from build123d import *

# Parameters (mm, degrees)
F1_DEPTH    = 112
F2_R        = 25
F3_DEPTH    = 185
F2_R_2      = 31.5
F5_DEPTH    = 184
F6_DEPTH    = 95
F7_W        = 48
F7_H        = 100
F8_DEPTH    = 159
F9_R        = 5.5
F10_DEPTH   = 39.1
F9_R_2      = 1.5
F11_DEPTH   = 154.4
F12_SIZE2   = 32
F12_SIZE    = 20
F12_2_SIZE2 = 32
F12_2_SIZE  = 20


with BuildPart() as f1:
    # F0 (on Front) → F1 (new body)
    with BuildSketch(Plane.XZ):
        with BuildLine():
            ThreePointArc((-59.7957043946, -22.8214863997), (-55.1094128936, -34.1351948987), (-43.7957043946, -38.8214863997))
            Line((-43.7957043946, -38.8214863997), (19.2042956054, -38.8214863997))
            ThreePointArc((19.2042956054, -38.8214863997), (30.5180041044, -34.1351948987), (35.2042956054, -22.8214863997))
            Line((35.2042956054, -22.8214863997), (35.2042956054, 103.1785136003))
            Line((35.2042956054, 103.1785136003), (29.2042956054, 103.1785136003))
            Line((29.2042956054, 103.1785136003), (29.2042956054, 87.1785136003))
            Line((29.2042956054, 87.1785136003), (29.2042956054, -23.8214863997))
            ThreePointArc((29.2042956054, -23.8214863997), (26.5682566361, -30.1854474304), (20.2042956054, -32.8214863997))
            Line((20.2042956054, -32.8214863997), (-44.7957043946, -32.8214863997))
            ThreePointArc((-44.7957043946, -32.8214863997), (-51.1596654253, -30.1854474304), (-53.7957043946, -23.8214863997))
            Line((-53.7957043946, -23.8214863997), (-53.7957043946, 86.1785136003))
            Line((-53.7957043946, 86.1785136003), (-59.7957043946, 86.1785136003))
            Line((-59.7957043946, 86.1785136003), (-59.7957043946, -22.8214863997))
        make_face()
    extrude(amount=F1_DEPTH)

    # F2 (on face) → F3 (cut)
    with BuildSketch(Plane.YZ.offset(35.2042956054)):
        with Locations((-56, 47.1785136003)):
            Circle(F2_R)
    extrude(amount=-F3_DEPTH, mode=Mode.SUBTRACT)

    # F2 (on face) → F5 (cut)
    with BuildSketch(Plane.YZ.offset(35.2042956054)):
        with Locations((-56, 47.1785136003)):
            Circle(F2_R_2)
        with Locations((-56, 47.1785136003)):
            Circle(F2_R, mode=Mode.SUBTRACT)
    extrude(amount=-F5_DEPTH, mode=Mode.SUBTRACT)

    # F2 (on face) → F6 (join)
    with BuildSketch(Plane.YZ.offset(35.2042956054)):
        with Locations((-56, 47.1785136003)):
            Circle(F2_R_2)
        with Locations((-56, 47.1785136003)):
            Circle(F2_R, mode=Mode.SUBTRACT)
    extrude(amount=-F6_DEPTH)

    # F7 (on offset) → F8 (cut)
    with BuildSketch(Plane.XZ.offset(137)):
        with Locations((-11.7957043946, 29.1785136003)):
            Rectangle(F7_W, F7_H)
    extrude(amount=-F8_DEPTH, mode=Mode.SUBTRACT)

    # F9 (on face) → F10 (cut)
    with BuildSketch(Plane.YZ.offset(35.2042956054)):
        with Locations((-83, 92.1785136003)):
            Circle(F9_R)
        with Locations((-29, 92.1785136003)):
            Circle(F9_R)
        with Locations((-95, 7.1785136003)):
            Circle(F9_R)
        with Locations((-17, 7.1785136003)):
            Circle(F9_R)
    extrude(amount=-F10_DEPTH, mode=Mode.SUBTRACT)

    # F9 (on face) → F11 (cut)
    with BuildSketch(Plane.YZ.offset(35.2042956054)):
        with Locations((-31.751288694, 33.2468845546)):
            Circle(F9_R_2)
        with Locations((-80.248711306, 33.2468845546)):
            Circle(F9_R_2)
        with BuildLine():
            ThreePointArc((-56, 73.7468845546), (-54.9393398282, 74.1862243828), (-54.5, 75.2468845546))
            ThreePointArc((-54.5, 75.2468845546), (-57.0606601718, 76.3075447264), (-56, 73.7468845546))
        make_face()
    extrude(amount=-F11_DEPTH, mode=Mode.SUBTRACT)

    # F12
    f12_edges = [f1.edges().sort_by_distance(p)[0] for p in [
        (-56.795704, 0, 86.178514),
        (-56.795704, -112, 86.178514),
    ]]
    f12_side = f1.faces().sort_by_distance((-56.795704, -56, 86.178514))[0]
    chamfer(f12_edges, length=F12_SIZE, length2=F12_SIZE2, reference=f12_side)

    # F12#2
    f12_2_edges = [f1.edges().sort_by_distance(p)[0] for p in [
        (32.204296, 0, 103.178514),
        (32.204296, -112, 103.178514),
    ]]
    f12_2_side = f1.faces().sort_by_distance((32.204296, -56, 103.178514))[0]
    chamfer(f12_2_edges, length=F12_2_SIZE, length2=F12_2_SIZE2, reference=f12_2_side)


solid = f1.part
Source: CAD feature listing. Evaluate the final solid. Frame: model axes, mm. A direction names the side the tool comes from. Coordinates: 2 decimals unless noted, no trailing zeros. Loops run counter-clockwise (first coordinate to the right, second up) from the corner with the lowest first, then second, coordinate; pieces in that order, holes last. Notation, with made-up numbers: (79, 27.5) - (99, 27.5) arc R11 cw to (99, 41.5) - close; hole circle Ø9 at (30.25, -17.5). An arc over 180 degrees is marked (long way). Return JSON: item names as keys, results as strings.
Q1. Section C-C, the plane y = -95. Return loops of the section in (x, z), plus the area to 3 significant figures.
Results:
{"outline": "(-59.8, -22.82) arc R16 ccw to (-43.8, -38.82) - (19.2, -38.82) arc R16 ccw to (35.2, -22.82) - (35.2, 1.68) - (29.2, 1.68) - (29.2, -23.82) arc R9 cw to (20.2, -32.82) - (-44.8, -32.82) arc R9 cw to (-53.8, -23.82) - (-53.8, 81.38) - (-59.8, 81.38) - close; (29.2, 12.68) - (35.2, 12.68) - (35.2, 98.38) - (29.2, 98.38) - close", "area": "1,900 mm2"}
Q2. Contact query for flat-ended pins moving along their axis: P1, Ø6, axis at x = -43, z = 43, coming from the -Y side; P2, Ø1, axis at x = -37.5, y = -74.5, coming from the +Z side; P3, Ø2.5, axis at y = -31.75, z = 33.25, coming from the +X side; P4, Ø10, axis at y = -17, z = 7.18, coming from the +X side. Output: stop coordinate, or through.
Results:
{"P1": "y = -87.48", "P2": "z = 73.03", "P3": "through", "P4": "x = -53.8"}
Q3. Section A-A, the plane z = -1. Return loops of the section in (x, y).
Results:
{"outline": "(-59.8, -112) - (-53.8, -112) - (-53.8, 0) - (-59.8, 0) - close; (29.2, -112) - (35.2, -112) - (35.2, 0) - (29.2, 0) - close"}
Q4. Material intervals for line 1 along X through (y, z) = (-69.5, 25.5); line 2 along X through (y, z) = (-5, 47); line 3 along Z through (x, y) = (-42.5, -66.5), sorted ascending.
Results:
{"line 1": "-59.8 to -35.8, 12.2 to 35.2", "line 2": "-59.8 to -53.8, 29.2 to 35.2", "line 3": "-38.82 to -32.82, 17.48 to 24.49, 69.87 to 76.88"}
Q5. Section D-D, the plane z = 40. Return loops of the section in (x, y), plus the area to 3 significant figures.
Results:
{"outline": "(-59.8, -112) - (-53.8, -112) - (-53.8, -86.67) - (-35.8, -86.67) - (-35.8, -79.95) - (-59.8, -79.95) - close; (-59.8, -32.05) - (-35.8, -32.05) - (-35.8, -25.33) - (-53.8, -25.33) - (-53.8, 0) - (-59.8, 0) - close; (12.2, -86.67) - (29.2, -86.67) - (29.2, -112) - (35.2, -112) - (35.2, -79.95) - (12.2, -79.95) - close; (12.2, -32.05) - (35.2, -32.05) - (35.2, 0) - (29.2, 0) - (29.2, -25.33) - (12.2, -25.33) - close", "area": "1,240 mm2"}
Q6. Access query for faces 4 (the flat face through (-56.754, -102.14, 69.955)), 5 (the flat face through (-12, -55, -32.821)), 6 (the flat face through (-57, -55, 86.179)). Directions: +Z, -Z, +X, -X, +Y, -Y. A direction counts if a zero-diameter tool reaches every point of the face in a straight line with its end or side. Return the directions, or none.
Results:
{"face 4": "+Z, -X, -Y", "face 5": "+Y, -Y", "face 6": "+Z, -X, +Y, -Y"}
Q7. Mould query, pull axis Z, two halves, no side actions, for faces 1 (the flat face through (-59.796, -55, 20)), 2 (the cylindrical face through (32.25, -11.92, 5.07)), 3 (the flat face through (32.246, -9.86, 86.955)). Classes: released by +Z, released by -Z, zero draft, split by the parting line, or undercut.
Results:
{"face 1": "zero draft", "face 2": "undercut", "face 3": "released by +Z"}
Q8. Section B-B, the plane x = 25.5. Return loops of the section in (y, z), plus the area to 3 significant figures.
Results:
{"outline": "(-112, -37.53) - (0, -37.53) - (0, -31.1) - (-112, -31.1) - close; circle Ø63 at (-56, 47.18); hole circle Ø3 at (-80.25, 33.25); hole circle Ø50 at (-56, 47.18); hole circle Ø3 at (-56, 75.25); hole circle Ø3 at (-31.75, 33.25)", "area": "1,850 mm2"}
